Input: part model. Units: mm. Frame: model coordinates. Round coordinates to 2 decimals unless told otherwise and drop trailing zeros. Order: outer loops, then holes, each group sorted by start corner. A loop starts at its lowest first (then second) coordinate and runs counter-clockwise, first axis right, second up. Notation, with made-up numbers: (34, 17) -> (76, 17) arc R22 cw to (76, 45) -> close; hole circle Ø4 at (1.25, 57.25). An arc over 180 degrees is marked (long way). Use a Markdown table: item, result.
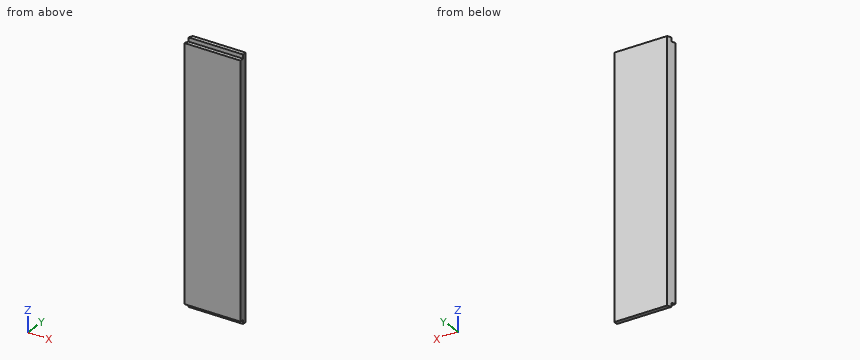
from build123d import *

# Parameters (mm, degrees)
BOSS_EXTRUDE1_DEPTH = 406.4
SKETCH2_W           = 89.154
SKETCH2_H           = 6.35
CUT_EXTRUDE1_DEPTH  = 6.35


with BuildPart() as part:
    # Sketch1 → Boss-Extrude1 (new body)
    with BuildSketch(Plane.XY):
        Polygon((0, 0), (5.260512242, 12.7), (89.154, 12.7), (89.154, 0), align=None)
    extrude(amount=BOSS_EXTRUDE1_DEPTH)

    # Sketch2 → Cut-Extrude1 (cut)
    with BuildSketch(Plane.XZ):
        with Locations((44.577, 3.175)):
            Rectangle(SKETCH2_W, SKETCH2_H)
        with Locations((44.577, 403.225)):
            Rectangle(SKETCH2_W, SKETCH2_H)
    extrude(amount=-CUT_EXTRUDE1_DEPTH, mode=Mode.SUBTRACT)


solid = part.part
1) Contact query for flat-ended pins moving along their axis: P1, Ø3, axis at x = 62.5, z = 2, coming from the -Y side; P2, Ø1.9, axis at x = 36.5, y = 2.5, coming from the -Z side; P3, Ø3, axis at x = 33, y = 2, coming from the +Z side. Output: stop coordinate, or through.
Answer key:
| item | result |
|---|---|
| P1 | stops at y = 6.35 |
| P2 | stops at z = 6.35 |
| P3 | stops at z = 400.05 |
2) Ray query, probe 1 along Z at (x, y) = (29, 6.25); probe 2 along X at (y, z) = (6.5, 87); probe 3 along X at (y, z) = (10.5, 39.5). Return the intervals inside material, ascending.
Answer key:
| item | result |
|---|---|
| probe 1 | z = 6.35 to 400.05 |
| probe 2 | x = 2.69 to 89.15 |
| probe 3 | x = 4.35 to 89.15 |
3) Cut plane B-B on z = 103.5. Return loops of the section in (x, y), and give its area (3 significant figures).
Answer key:
| item | result |
|---|---|
| outline | (0, 0) -> (89.15, 0) -> (89.15, 12.7) -> (5.26, 12.7) -> close |
| area | 1,100 mm^2 |
4) Cut plane C-C on y = 9.5. Return loops of the section in (x, z).
Answer key:
| item | result |
|---|---|
| outline | (3.94, 0) -> (89.15, 0) -> (89.15, 406.4) -> (3.94, 406.4) -> close |
5) Cut plane A-A on x = 74.5. Return loops of the section in (y, z), and give its area (3 significant figures).
Answer key:
| item | result |
|---|---|
| outline | (0, 6.35) -> (6.35, 6.35) -> (6.35, 0) -> (12.7, 0) -> (12.7, 406.4) -> (6.35, 406.4) -> (6.35, 400.05) -> (0, 400.05) -> close |
| area | 5,080 mm^2 |
